Could you check a few things on this drawing? It's one solid part, dimensions in mm from its lowest x, y, z. Give positions to 0.01 mm unless a question says otherwise; leave off trailing zeros. Loops run counter-clockwise (first coordinate to the right, second up) from the corner with the lowest first, then second, coordinate; pieces in that order, holes last. Notation, with made-up numbers: (-34.5, 84.25) - (-1.5, 84.25) arc R38 ccw to (-1.5, 122.25) - close; hole circle Ø1 at (-3.5, -25). An arc over 180 degrees is marked (long way). Use a Markdown table: item, result.
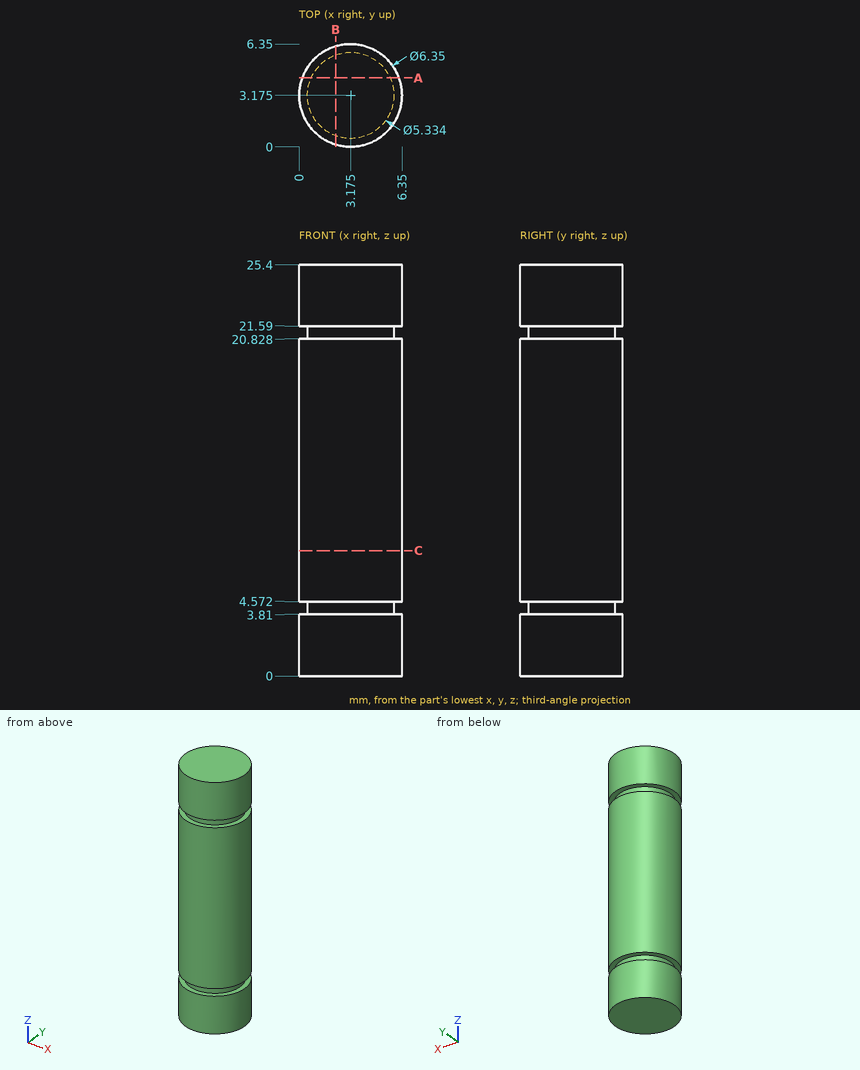
(1) Will this pin go through, and if not, where does the flat tip stop? pin 1 (2 mm diameter, centred on y = 4.5, z = 20.5, fed in from +X).
A:
| item | result |
|---|---|
| pin 1 | x = 6.33 |
(2) Suppose I cut it at A-A on y = 4.25. Write out the boundary of the cut face in (x, z).
A:
| item | result |
|---|---|
| outline | (0.19, 0) - (6.16, 0) - (6.16, 3.81) - (5.62, 3.81) - (5.62, 4.57) - (6.16, 4.57) - (6.16, 20.83) - (5.62, 20.83) - (5.62, 21.59) - (6.16, 21.59) - (6.16, 25.4) - (0.19, 25.4) - (0.19, 21.59) - (0.73, 21.59) - (0.73, 20.83) - (0.19, 20.83) - (0.19, 4.57) - (0.73, 4.57) - (0.73, 3.81) - (0.19, 3.81) - close |
(3) Suppose I cut it at B-B on x = 2.25. Write out the boundary of the cut face in (y, z), plus the area to 3 significant figures.
A:
| item | result |
|---|---|
| outline | (0.14, 0) - (6.21, 0) - (6.21, 3.81) - (5.68, 3.81) - (5.68, 4.57) - (6.21, 4.57) - (6.21, 20.83) - (5.68, 20.83) - (5.68, 21.59) - (6.21, 21.59) - (6.21, 25.4) - (0.14, 25.4) - (0.14, 21.59) - (0.67, 21.59) - (0.67, 20.83) - (0.14, 20.83) - (0.14, 4.57) - (0.67, 4.57) - (0.67, 3.81) - (0.14, 3.81) - close |
| area | 153 mm2 |
(4) Suppose I cut it at C-C on z = 7.75. Write out the boundary of the cut face in (x, y) (3 decimals), plus the area to 3 significant figures.
A:
| item | result |
|---|---|
| outline | circle Ø6.35 at (3.175, 3.175) |
| area | 31.7 mm2 |
(5) If I drill on line 1 (Z direction, x = 2.75, y = 0.5); line 2 (X direction, y = 3, z = 8), over which ranges is the centre line in solid material (lowest first)?
A:
| item | result |
|---|---|
| line 1 | 0 to 3.81, 4.57 to 20.83, 21.59 to 25.4 |
| line 2 | 0 to 6.35 |
